For this review, use the dimensioned drawing (mm, ordinates from the lowest corner) and the shaded views. Round coordinates to 2 decimals unless told otherwise and drop trailing zeros. Loops run counter-clockwise (first coordinate to the right, second up) from the corner with the lowest first, then second, coordinate; pieces in that order, holes last. Notation, with made-up numbers: (-25, -18) -> (33, -18) arc R21 cw to (33, 15) -> close; hole circle Ø5 at (8, -38.5). An arc over 180 degrees is marked (long way). Use one line per item in the form item = value. Start each with the question number.
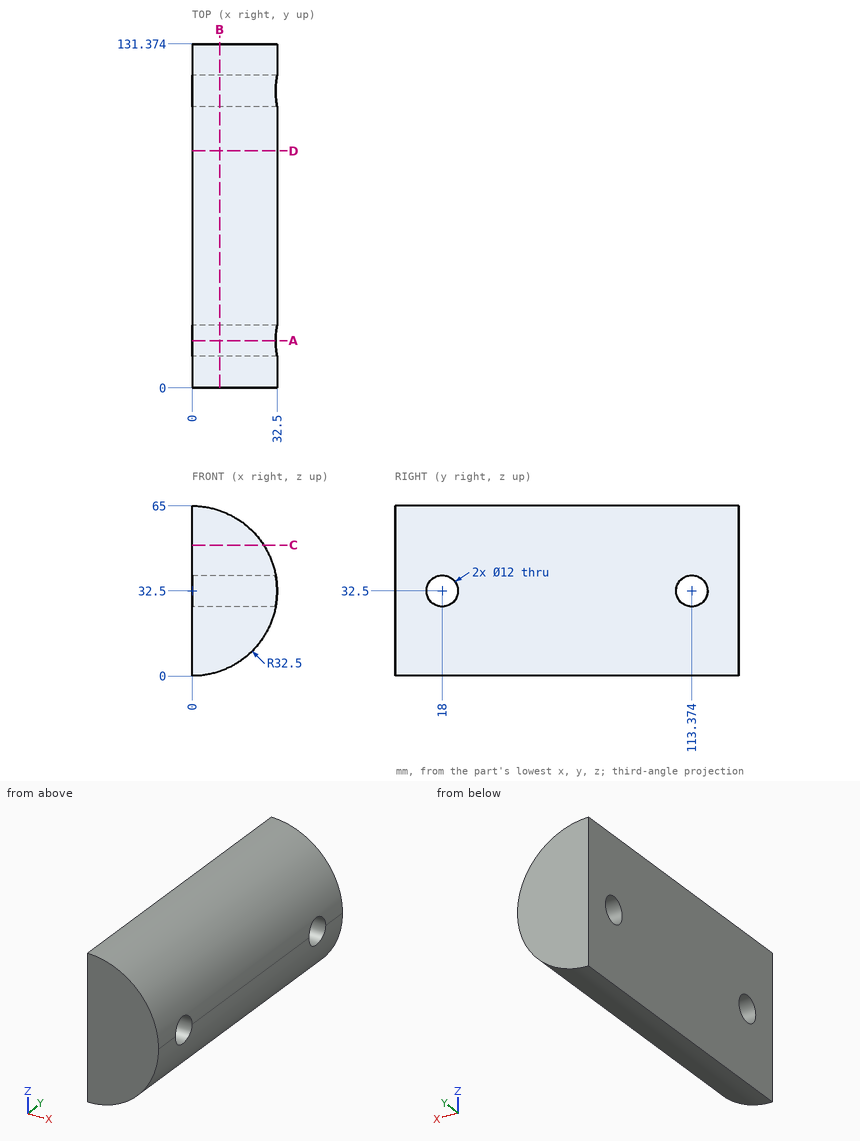
Item 1: For P1, Ø3, axis at x = 27, y = 16, coming from the +Z side; P2, Ø2, axis at x = 27.5, y = 30.5, coming from the +Z side (1 decimal); P3, Ø3, axis at x = 3.5, y = 80, coming from the +Z side, all flat-tipped, find the tip position at first contact; note any pin that passes through.
Item 2: Take a section at D-D on y = 90.5. Give the boundary of the cut face in (x, z), plus the area to 3 significant figures.
Item 3: Take a section at A-A on y = 18. Give the boundary of the cut face in (x, z), plus the area to 3 significant figures.
Item 4: Take a section at C-C on z = 50. Give the boundary of the cut face in (x, y).
Item 5: Take a section at B-B on x = 10.5. Give the boundary of the cut face in (y, z).
Item 6: Wall thickness on line 1 (Y direction, x = 17, z = 32.5); line 2 (Y direction, x = 7.5, z = 34) (1 decimal); line 3 (X direction, y = 123, z = 28.5): over which ranges is each line inside the solid? List them lowest first.
Results:
q1.P1 = 52.65
q1.P2 = 51.3
q1.P3 = 64.94
q2.outline = (0, 0) arc R32.5 ccw to (0, 65) -> close
q2.area = 1,660 mm2
q3.outline = (0, 0) arc R32.5 ccw to (31.94, 26.5) -> (0, 26.5) -> close; (0, 38.5) -> (31.94, 38.5) arc R32.5 ccw to (0, 65) -> close
q3.area = 1,270 mm2
q4.outline = (0, 0) -> (27.39, 0) -> (27.39, 131.37) -> (0, 131.37) -> close
q5.outline = (0, 1.74) -> (131.37, 1.74) -> (131.37, 63.26) -> (0, 63.26) -> close; hole circle Ø12 at (18, 32.5); hole circle Ø12 at (113.37, 32.5)
q6.line_1 = 0 to 12, 24 to 107.37, 119.37 to 131.37
q6.line_2 = 0 to 12.2, 23.8 to 107.6, 119.2 to 131.4
q6.line_3 = 0 to 32.25
